from build123d import *

# Parameters (mm, degrees)
SKETCH1_R           = 2.6
BOSS_EXTRUDE1_DEPTH = 304.8
FILLET1_R           = 2


with BuildPart() as part:
    # Sketch1 → Boss-Extrude1 (new body)
    with BuildSketch(Plane.XY):
        Polygon((-3.9, 2.910050506), (-6.179949494, 5.19), (-8.15, 5.19), (-8.15, 3.1), (-10, 3.1), (-10, 10), (-3.1, 10), (-3.1, 8.15), (-5.19, 8.15), (-5.19, 6.179949494), (-2.910050506, 3.9), (2.910050506, 3.9), (5.19, 6.179949494), (5.19, 8.15), (3.1, 8.15), (3.1, 10), (10, 10), (10, 3.1), (8.15, 3.1), (8.15, 5.19), (6.179949494, 5.19), (3.9, 2.910050506), (3.9, -2.910050506), (6.179949494, -5.19), (8.15, -5.19), (8.15, -3.1), (10, -3.1), (10, -10), (3.1, -10), (3.1, -8.15), (5.19, -8.15), (5.19, -6.179949494), (2.910050506, -3.9), (-2.910050506, -3.9), (-5.19, -6.179949494), (-5.19, -8.15), (-3.1, -8.15), (-3.1, -10), (-10, -10), (-10, -3.1), (-8.15, -3.1), (-8.15, -5.19), (-6.179949494, -5.19), (-3.9, -2.910050506), align=None)
        Circle(SKETCH1_R, mode=Mode.SUBTRACT)
    extrude(amount=-BOSS_EXTRUDE1_DEPTH)

    # Fillet1
    fillet1_edges = [part.edges().sort_by_distance(p)[0] for p in [
        (-10, 10, -152.4),
        (10, 10, -152.4),
        (10, -10, -152.4),
        (-10, -10, -152.4),
    ]]
    fillet(fillet1_edges, radius=FILLET1_R)


solid = part.part
Part model, mm, in its own coordinate system. A direction names the side the tool comes from. Coordinates: 2 decimals unless noted, no trailing zeros. Order: outer loops, then holes, each group sorted by start corner. A loop starts at its lowest first (then second) coordinate and runs counter-clockwise, first axis right, second up. Notation, with made-up numbers: (66.25, 50.25) - (79.25, 50.25) arc R38 cw to (79.25, 89.25) - close; hole circle Ø6 at (67.5, -1.5). An arc over 180 degrees is marked (long way). Use CSV: the item, a comma, the result in double quotes.
Item 1: Saw through at A-A on y = 0. Give the cut face in (x, z).
Solved:
outline,"(-3.9, -304.8) - (-2.6, -304.8) - (-2.6, 0) - (-3.9, 0) - close; (2.6, -304.8) - (3.9, -304.8) - (3.9, 0) - (2.6, 0) - close"
Item 2: Probe probe 1 along Y at (x, z) = (8.25, -278.5); probe 2 along X at (y, z) = (-7, -207.5); probe 3 along Y at (x, z) = (4.5, -124). List the from-to ranges inside material, lowest first.
Solved:
probe 1,"y = -9.98 to -3.1, 3.1 to 9.98"
probe 2,"x = -10 to -5.19, 5.19 to 10"
probe 3,"y = -10 to -8.15, -5.49 to -3.51, 3.51 to 5.49, 8.15 to 10"
Item 3: Drop flat-ended pins along their axis: P1, Ø12, axis at y = -2.5, z = -145.5, coming from the +X side; P2, Ø0.9, axis at y = 9, z = -199, coming from the +X side; P3, Ø3, axis at y = -1, z = -222, coming from the -X side; P4, Ø1.5, axis at y = 9.5, z = -150, coming from the -X side. Give the stop position or say it passes through.
Solved:
P1,"stops at x = 10"
P2,"stops at x = 9.92"
P3,"stops at x = -3.9"
P4,"stops at x = -9.85"
Item 4: 3-axis set-ups, long thin cutter, end or side, ignore diameter. For faces 1 (the face through (0, 3.9, -150)), 2 (the face through (3.9, 0, -150)), 3 (the face through (-3.9, 0, -150)): which of +Z, -Z, +X, -X, +Y, -Y reach the whole face in a straight line?
Solved:
face 1,"+Z, -Z, +Y"
face 2,"+Z, -Z, +X"
face 3,"+Z, -Z, -X"
Item 5: Mould opens along X. For faces 4 (the face through (-10, -6, -150)), 5 (the face through (-0.338, 2.578, -150.266)), 6 (the face through (0, -3.9, -150)), 7 (the face through (10, -6, -150)) say: +X half, -X half, draft (parallel to the pull), parting line (faces both ways), or undercut.
Solved:
face 4,"-X half"
face 5,"undercut"
face 6,"undercut"
face 7,"+X half"
